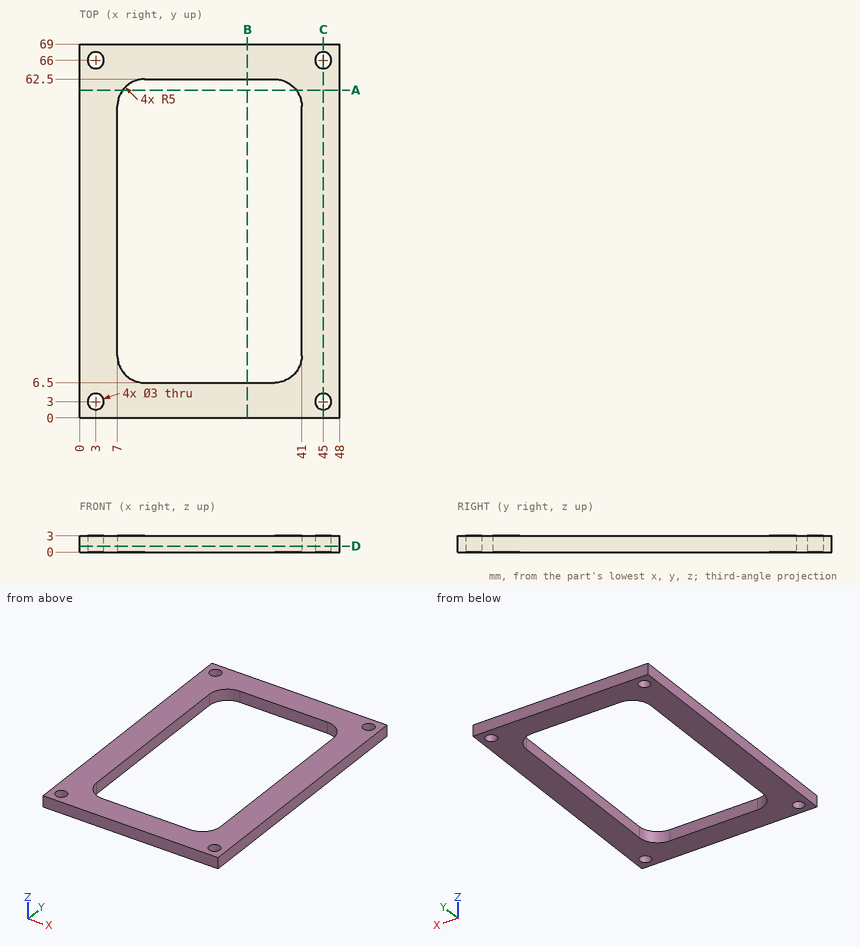
Study the drawing (mm; zero at the part's minimum x, y, z) and answer. Give positions to 0.01 mm unless a question says otherwise; leave off trailing zeros. Write each loop counter-clockwise with the first axis right and the second up, starting at its lowest first coordinate (ties: lowest second). Pieces come first, ordered by that corner, then holes. Notation, with made-up numbers: (56, 7.5) -> (106, 7.5) arc R25 ccw to (106, 34.5) -> close; hole circle Ø7 at (33.5, 27.25). An arc over 180 degrees is marked (long way). Answer as a JSON object with one key per item and string values. Group by question number.
1) Consider L1, parallel to Y at x = 3, z = 1.25; L2, parallel to X at y = 66, z = 1.4; L3, parallel to X at y = 26, z = 0.65. Determine where each line is inside the solid, lowest interval first. Write a range as from..to.
2) Find section C-C (x = 45). Write down the section's boundary in (y, z).
3) Find section B-B (x = 31). Write down the section's boundary in (y, z).
4) Find section D-D (z = 1.1). Write down the section's boundary in (x, y).
5) Find section A-A (y = 60.5). Write down the section's boundary in (x, z), and give its area (3 significant figures).
Values follow:
{
 "1": {"L1": "y = 0..1.5, 4.5..64.5, 67.5..69", "L2": "x = 0..1.5, 4.5..43.5, 46.5..48", "L3": "x = 0..7, 41..48"},
 "2": {"outline": "(0, 0) -> (1.5, 0) -> (1.5, 3) -> (0, 3) -> close; (4.5, 0) -> (64.5, 0) -> (64.5, 3) -> (4.5, 3) -> close; (67.5, 0) -> (69, 0) -> (69, 3) -> (67.5, 3) -> close"},
 "3": {"outline": "(0, 0) -> (6.5, 0) -> (6.5, 3) -> (0, 3) -> close; (62.5, 0) -> (69, 0) -> (69, 3) -> (62.5, 3) -> close"},
 "4": {"outline": "(0, 0) -> (48, 0) -> (48, 69) -> (0, 69) -> close; hole circle Ø3 at (3, 3); hole circle Ø3 at (3, 66); hole (7, 11.5) arc R5 ccw to (12, 6.5) -> (36, 6.5) arc R5 ccw to (41, 11.5) -> (41, 57.5) arc R5 ccw to (36, 62.5) -> (12, 62.5) arc R5 ccw to (7, 57.5) -> close; hole circle Ø3 at (45, 3); hole circle Ø3 at (45, 66)"},
 "5": {"outline": "(0, 0) -> (8, 0) -> (8, 3) -> (0, 3) -> close; (40, 0) -> (48, 0) -> (48, 3) -> (40, 3) -> close", "area": "48.0 mm2"}
}
